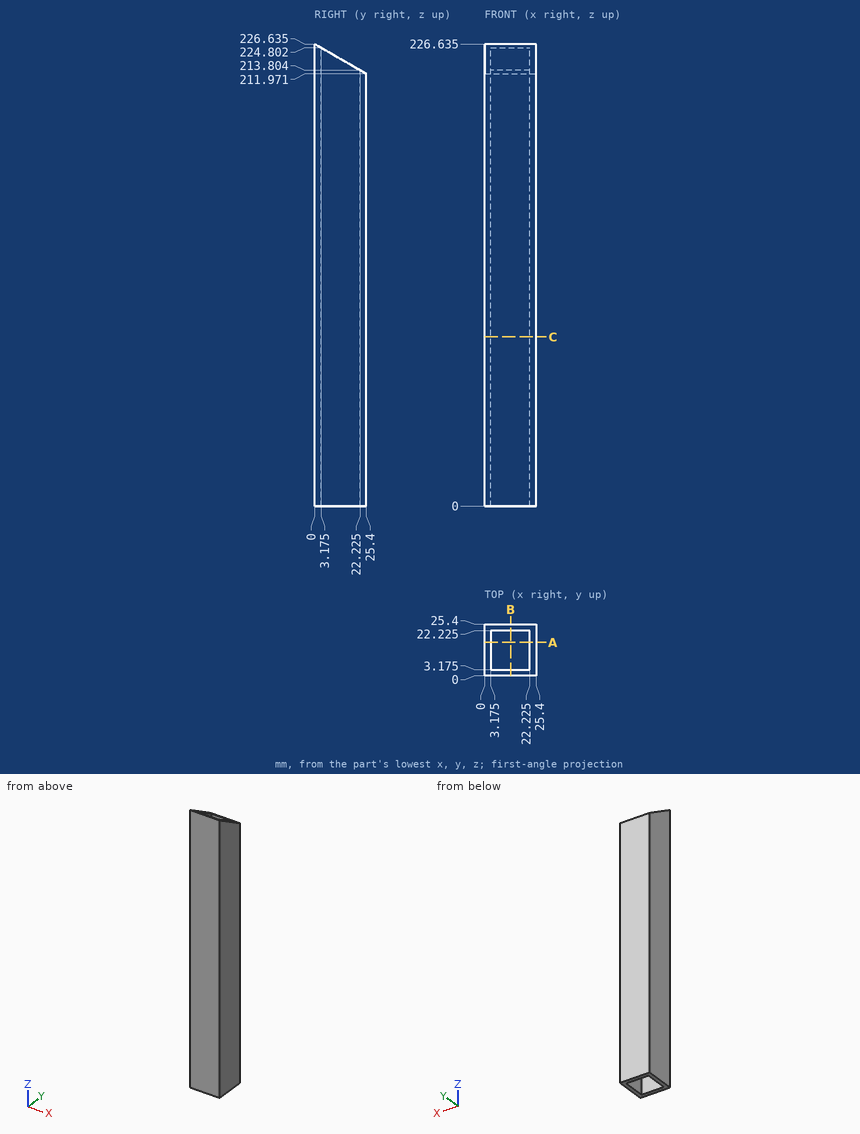
Could you check a few things on this drawing? It's one solid part, dimensions in mm from its lowest x, y, z. Coordinates: 2 decimals unless noted, no trailing zeros. Order: outer loops, then holes, each group sorted by start corner. A loop starts at its lowest first (then second) coordinate and runs counter-clockwise, first axis right, second up. Notation, with made-up numbers: (0, 53) -> (34, 53) arc R34 cw to (34, 85) -> close; hole circle Ø10 at (68.25, -15.5). An arc over 180 degrees is marked (long way). One line per item, written item: value. Start each with the question number.
1) If I drill on L1, parallel to Y at x = 15, z = 111.5 (1 decimal); L2, parallel to Y at x = 4.25, z = 215 (1 decimal), over which ranges is the centre line in solid material (lowest first)? Write a range as [from, to].
2) I'm going to push flat-ended pins straight in: pin 1 (3 mm diameter, centred on x = 21, y = 21, fed in from +Z); pin 2 (1.5 mm diameter, centred on x = 19.5, y = 6.5, fed in from +Z); pin 3 (6 mm diameter, centred on x = 3.5, y = 18, fed in from +Z) (1 decimal). Where does each tip first touch, or does it pass through?
3) Imagine slicing it at A-A on y = 16.5. List the corners of the cut face in (x, z) for me (1 decimal), plus the area to 3 significant figures.
4) Imagine slicing it at B-B on x = 12.75. List the corners of the cut face in (y, z) for me (1 decimal).
5) Imagine slicing it at C-C on z = 83. List the corners of the cut face in (x, y) for me (1 decimal).
Answer list:
1. L1: y = [0, 3.2], [22.2, 25.4]
1. L2: y = [0, 3.2]
2. pin 1: stops at z = 215.01
2. pin 2: passes through
2. pin 3: stops at z = 218
3. outline: (0, 0) -> (3.2, 0) -> (3.2, 217.1) -> (0, 217.1) -> close; (22.2, 0) -> (25.4, 0) -> (25.4, 217.1) -> (22.2, 217.1) -> close
3. area: 1,380 mm2
4. outline: (0, 0) -> (3.2, 0) -> (3.2, 224.8) -> (0, 226.6) -> close; (22.2, 0) -> (25.4, 0) -> (25.4, 212) -> (22.2, 213.8) -> close
5. outline: (0, 0) -> (25.4, 0) -> (25.4, 25.4) -> (0, 25.4) -> close; hole (3.2, 3.2) -> (22.2, 3.2) -> (22.2, 22.2) -> (3.2, 22.2) -> close
